For this review, take the finished solid that the model builds, in its own axes (mm). Face numbers are marked on the shaded views. A direction names the side the tool comes from. Round coordinates to 2 decimals unless told otherwise and drop trailing zeros. Write each loop counter-clockwise with the first axis right and the second up, starting at its lowest first coordinate (ties: lowest second). Pieces come first, ordered by that corner, then holes. Notation, with made-up numbers: (56, 51.25) -> (67, 51.25) arc R33 cw to (67, 85.25) -> close; hole circle Ø5 at (-25.75, 38.5). An arc over 180 degrees is marked (long way). Write each question's results on one line, items separated by ' | '. Start each with the question number.
Item 1: Tool access review of the marked faces 4 and 5: name each direction out of +Z, -Z, +X, -X, +Y, -Y from which nothing blocks a thin tool from reaching the whole face with its end or side.
Item 2: To check wall thickness, follow line 1 along X through (y, z) = (90.5, 3.5) (3 decimals); line 2 along Z through (x, y) = (-13, 11) (1 decimal). State the ranges of each line that lie inside material, in increasing order.
Item 3: Add section B-B (y = 58). State the section outline as (x, z) points (1 decimal).
Item 4: The part is to be moulded in two halves that separate along Z. For the marked faces 1, 2 and 3, say which applies: +Z half, -Z half, draft (parallel to the pull), parting line (faces both ways), or undercut.
Item 5: Add section A-A (x = 0.5). State the section outline as (y, z) points (3 decimals).
Item 6: Add section C-C (z = -8.5). State the section outline as (x, y) points (3 decimals), plus the area to 3 significant figures.
Autodesk Inventor part; units mm, degrees
ref_plane "YZ Plane" through (0, 0, 0) normal (1, 0, 0) x (0, 1, 0)
ref_plane "XZ Plane" through (0, 0, 0) normal (0, 1, 0) x (-1, 0, 0)
ref_plane "XY Plane" through (0, 0, 0) normal (0, 0, 1) x (1, 0, 0)
sketch "Sketch1" plane through (0, 0, 0) normal (0, 1, 0) x (-1, 0, 0)
  line L0 (12.7, 12.7) -> (-12.7, 12.7)
  line L1 (-12.7, 12.7) -> (-12.7, -12.7)
  line L2 (-12.7, -12.7) -> (12.7, -12.7)
  line L3 (12.7, -12.7) -> (12.7, 12.7)
  line L4 (12.7, 12.7) -> (-12.7, -12.7) construction
  line L5 (-12.7, 12.7) -> (12.7, -12.7) construction
  line L6 (15.875, 15.875) -> (-15.875, 15.875)
  line L7 (-15.875, 15.875) -> (-15.875, -15.875)
  line L8 (-15.875, -15.875) -> (15.875, -15.875)
  line L9 (15.875, -15.875) -> (15.875, 15.875)
  line L10 (15.875, 15.875) -> (-15.875, -15.875) construction
  line L11 (-15.875, 15.875) -> (15.875, -15.875) construction
  point P0 (0, 0)
  dimension "d0" = 25.4
  dimension "d1" = 25.4
  dimension "d2" = 3.175
  dimension "d3" = 3.175
extrude "Extrusion1" add sketch "Sketch1" along normal blind 95.1992
sketch "Sketch2" plane through (15.875, 0, 15.875) normal (1, 0, 0) x (0, 0, -1)
  line L0 (15.875, 0) -> (15.875, 69.7992) construction
  line L1 (20.6375, 0) -> (20.6375, 69.7992)
  line L2 (11.1125, 69.7992) -> (11.1125, 0)
  arc A0 (11.1125, 0) -> (20.6375, 0) centre (15.875, 0) ccw
  arc A1 (20.6375, 69.7992) -> (11.1125, 69.7992) centre (15.875, 69.7992) ccw
  line L3 (0, 0) -> (31.75, 0)
  point P0 (15.875, 34.8996)
  dimension "d6" = 4.7625
  dimension "d7" = 69.7992
extrude "Extrusion2" cut sketch "Sketch2" against normal through all
sketch "Sketch3" plane through (-15.875, 0, 15.875) normal (0, 0, 1) x (1, 0, 0)
  line L0 (15.875, 0) -> (15.875, 95.1992) construction
  line L1 (28.575, 95.1992) -> (3.175, 95.1992) construction
  line L2 (0, 0) -> (31.75, 0) construction
  point P0 (15.875, 50.8)
  dimension "d10" = 50.8
properties part number "capForPost"
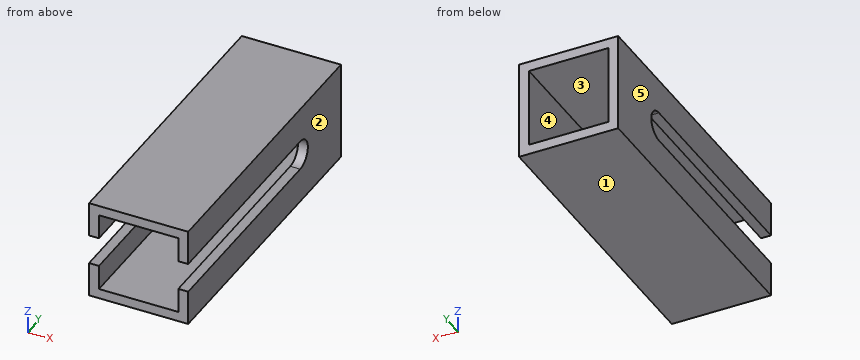
Responses:
1) face 4: +Y, -Y | face 5: +Z, -Z, -X, +Y, -Y
2) line 1: x = -15.875 to -12.7, 12.7 to 15.875 | line 2: z = -15.9 to -4.8, 4.8 to 15.9
3) outline: (-15.9, -15.9) -> (15.9, -15.9) -> (15.9, -4.8) -> (12.7, -4.8) -> (12.7, -12.7) -> (-12.7, -12.7) -> (-12.7, -4.8) -> (-15.9, -4.8) -> close; (-15.9, 4.8) -> (-12.7, 4.8) -> (-12.7, 12.7) -> (12.7, 12.7) -> (12.7, 4.8) -> (15.9, 4.8) -> (15.9, 15.9) -> (-15.9, 15.9) -> close
4) face 1: -Z half | face 2: draft | face 3: undercut
5) outline: (0, -15.875) -> (95.199, -15.875) -> (95.199, -12.7) -> (0, -12.7) -> close; (0, 12.7) -> (95.199, 12.7) -> (95.199, 15.875) -> (0, 15.875) -> close
6) outline: (-15.875, 0) -> (-12.7, 0) -> (-12.7, 95.199) -> (-15.875, 95.199) -> close; (12.7, 0) -> (15.875, 0) -> (15.875, 95.199) -> (12.7, 95.199) -> close | area: 605 mm^2
